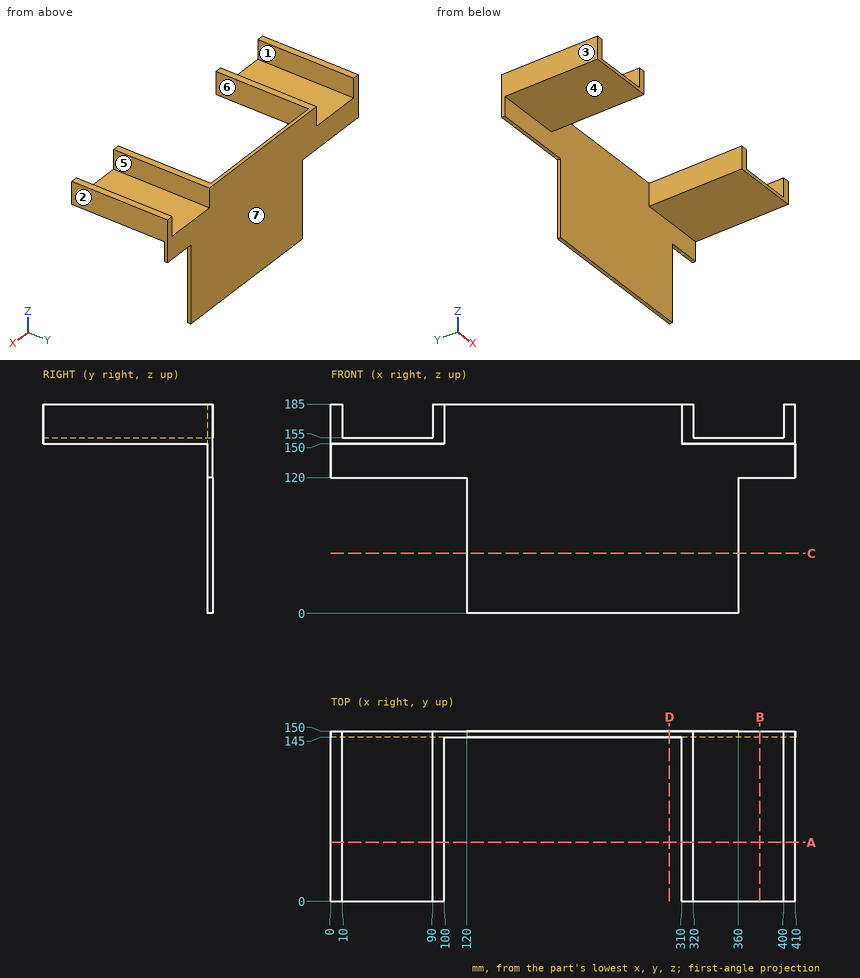
For this review, use the dimensioned drawing (mm, ordinates from the lowest corner) and the shaded views. A direction names the side the tool comes from. Coordinates: 2 decimals unless noted, no trailing zeros. Write each loop counter-clockwise with the first axis right and the second up, starting at its lowest first coordinate (ties: lowest second). Pieces come first, ordered by that corner, then holes. Notation, with made-up numbers: (3.25, 85.5) - (53.25, 85.5) arc R22 cw to (53.25, 115.5) - close; hole circle Ø6 at (-25, -10.5). An arc over 180 degrees is marked (long way). Answer in a Markdown table with one row per item. Add a question column.
Q1. Consider section D-D on x = 299. Give the boundary of the cut face in (y, z).
Q2. For the marked faces 4, 5, 6 and 7, list the 3-axis set-ups (+Z, -Z, +X, -X, +Y, -Y) from which the entire face can be reached by the end or side of a thin tool; tool diameter is ignored.
Q3. Consider section B-B on x = 379. Give the boundary of the cut face in (y, z).
Q4. Draft analysis for pull direction X (two halves, no side actions). For the marked faces 1, 2 and 3, state which applies: +X half, -X half, draft (parallel to the pull), parting line (faces both ways), or undercut.
Q5. To check wall thickness, follow line 1 along X through (y, z) = (63, 173); line 2 along Y through (x, z) = (373.5, 136); line 3 along Z through (x, y) = (22.5, 129.5). State the ranges of each line that lie inside material, in increasing order. Write a range as from..to.
Q6. Clearance check with flat-ended pins moving along their axes: pin 1 (24 mm diameter, centred on x = 42.5, y = 54.5, fed in from +Z); pin 2 (1.5 mm diameter, centred on y = 148, z = 61, fed in from -X); pin 3 (5.5 mm diameter, centred on x = 381.5, y = 147.5, fed in from -Z). State where each tip first meets the part, or that it passes through.
Q7. Consider section A-A on y = 52. Give the boundary of the cut face in (x, z), then the cut area to 3 significant figures.
Q8. Consider section C-C on z = 53. Give the boundary of the cut face in (x, y), then the cut area to 3 significant figures.
Answers below:
| question | item | result |
|---|---|---|
| 1 | outline | (145, 0) - (150, 0) - (150, 185) - (145, 185) - close |
| 2 | face 4 | -Z, +X, -X, -Y |
| 2 | face 5 | +Z, +Y, -Y |
| 2 | face 6 | +Z, -Z, -Y |
| 2 | face 7 | +Z, -Z, +X, -X, +Y |
| 3 | outline | (0, 150) - (145, 150) - (145, 120) - (150, 120) - (150, 155) - (0, 155) - close |
| 4 | face 1 | undercut |
| 4 | face 2 | +X half |
| 4 | face 3 | -X half |
| 5 | line 1 | 0..10, 90..100, 310..320, 400..410 |
| 5 | line 2 | 145..150 |
| 5 | line 3 | 150..155 |
| 6 | pin 1 | z = 155 |
| 6 | pin 2 | x = 120 |
| 6 | pin 3 | z = 120 |
| 7 | outline | (0, 150) - (100, 150) - (100, 185) - (90, 185) - (90, 155) - (10, 155) - (10, 185) - (0, 185) - close; (310, 150) - (410, 150) - (410, 185) - (400, 185) - (400, 155) - (320, 155) - (320, 185) - (310, 185) - close |
| 7 | area | 2,200 mm² |
| 8 | outline | (120, 145) - (360, 145) - (360, 150) - (120, 150) - close |
| 8 | area | 1,200 mm² |
